The model under review builds one solid part; all positions refer to its coordinate system, in mm. A direction names the side the tool comes from. Coordinates: 2 decimals unless noted, no trailing zeros. Write each loop counter-clockwise with the first axis right and the second up, starting at its lowest first coordinate (ties: lowest second). Pieces come first, ordered by that corner, then holes. Notation, with made-up numbers: (-27.5, 37.5) - (28.5, 37.5) arc R26 cw to (28.5, 73.5) - close; hole circle Ø3 at (63, 19). An arc over 180 degrees is marked (long way). Use one line per item in the form item = value. Start each with the question number.
```python
from build123d import *

# Parameters (mm, degrees)
SKETCH1_W           = 600
SKETCH1_H           = 600
BOSS_EXTRUDE1_DEPTH = 10
SKETCH2_W           = 20
SKETCH2_H           = 60
BOSS_EXTRUDE2_DEPTH = 130
SKETCH3_W           = 600
SKETCH3_H           = 600
SKETCH3_W_2         = 20
SKETCH3_H_2         = 60
BOSS_EXTRUDE3_DEPTH = 10
SKETCH4_OUTSIDE_W   = 774
SKETCH4_OUTSIDE_H   = 774
SKETCH4_OUTSIDE_W_2 = 600
SKETCH4_OUTSIDE_H_2 = 80
CUT_EXTRUDE1_DEPTH  = 10
SKETCH5_W           = 42
SKETCH5_H           = 42
CUT_EXTRUDE2_DEPTH  = 10


with BuildPart() as part:
    # Sketch1 → Boss-Extrude1 (new body)
    with BuildSketch(Plane(origin=(0, 0, 0), x_dir=(1, 0, 0), z_dir=(0, 1, 0))):
        Rectangle(SKETCH1_W, SKETCH1_H)
    extrude(amount=BOSS_EXTRUDE1_DEPTH)

    # Sketch2 → Boss-Extrude2 (add)
    with BuildSketch(Plane(origin=(0, 10, 0), x_dir=(1, 0, 0), z_dir=(0, 1, 0))):
        with Locations((-250, 0)):
            Rectangle(SKETCH2_W, SKETCH2_H)
        with Locations((250, 0)):
            Rectangle(SKETCH2_W, SKETCH2_H)
    extrude(amount=BOSS_EXTRUDE2_DEPTH)

    # Sketch3 → Boss-Extrude3 (add)
    with BuildSketch(Plane(origin=(0, 110, 0), x_dir=(1, 0, 0), z_dir=(0, 1, 0))):
        Rectangle(SKETCH3_W, SKETCH3_H)
        with Locations((-250, 0)):
            Rectangle(SKETCH3_W_2, SKETCH3_H_2, mode=Mode.SUBTRACT)
        with Locations((250, 0)):
            Rectangle(SKETCH3_W_2, SKETCH3_H_2, mode=Mode.SUBTRACT)
    extrude(amount=BOSS_EXTRUDE3_DEPTH)

    # Sketch4 outside → Cut-Extrude1 (cut)
    with BuildSketch(Plane(origin=(0, 120, 0), x_dir=(1, 0, 0), z_dir=(0, 1, 0))):
        Rectangle(SKETCH4_OUTSIDE_W, SKETCH4_OUTSIDE_H)
        Rectangle(SKETCH4_OUTSIDE_W_2, SKETCH4_OUTSIDE_H_2, mode=Mode.SUBTRACT)
    extrude(amount=-CUT_EXTRUDE1_DEPTH, mode=Mode.SUBTRACT)

    # Sketch5 → Cut-Extrude2 (cut)
    with BuildSketch(Plane(origin=(0, 120, 0), x_dir=(1, 0, 0), z_dir=(0, 1, 0))):
        with Locations((-40, 0)):
            Rectangle(SKETCH5_W, SKETCH5_H)
        with Locations((40, 0)):
            Rectangle(SKETCH5_W, SKETCH5_H)
    extrude(amount=-CUT_EXTRUDE2_DEPTH, mode=Mode.SUBTRACT)


solid = part.part
```
1. For P1, Ø2, axis at x = 174, z = 136, coming from the +Y side; P2, Ø22, axis at y = 132.5, z = -7.5, coming from the -X side; P3, Ø22, axis at x = 246.5, y = 80.5, coming from the +Z side, all flat-tipped, find the tip position at first contact; note any pin that passes through.
2. Take a section at A-A (y = 53.5). State the section outline as (x, z) points, plus the area to 3 significant figures.
3. Take a section at B-B (x = -217.5). State the section outline as (y, z) points, plus the area to 3 significant figures.
4. For faces 4 (the flat face through (250, 59, 30)), 5 (the flat face through (260, 59, 0)), 6 (the flat face through (240, 130, 0)), 7 (the flat face through (240, 59, 0)), 8 (the flat face through (260, 130, 0)), list the 3-axis set-ups (+Z, -Z, +X, -X, +Y, -Y) from which the entire face can be reached by the end or side of a thin tool; tool diameter is ignored.
5. Take a section at C-C (z = 131). State the section outline as (x, y) points.
6. For L1, parallel to Z at x = -77.5, y = 118; L2, parallel to X at y = 75, z = 16; L3, parallel to Y at x = 233, z = 20, list the stretches that pass through material, from the lowest coordinate up.
7. The part is to be moulded in two halves that separate along Y. For faces 1 (the flat face through (250, 140, 0)), 2 (the flat face through (-250, 130, -30)), 3 (the flat face through (-260, 59, 0)), say which applies: released by +Y, released by -Y, zero draft, split by the parting line, or undercut.
Returned:
q1.P1 = 10
q1.P2 = -260
q1.P3 = 30
q2.outline = (-260, -30) - (-240, -30) - (-240, 30) - (-260, 30) - close; (240, -30) - (260, -30) - (260, 30) - (240, 30) - close
q2.area = 2,400 mm²
q3.outline = (0, -300) - (10, -300) - (10, 300) - (0, 300) - close; (110, -40) - (120, -40) - (120, 40) - (110, 40) - close
q3.area = 6,800 mm²
q4.face_4 = +Z, +X, -X
q4.face_5 = +Z, -Z, +X
q4.face_6 = +Z, -Z, +Y
q4.face_7 = +Z, -Z
q4.face_8 = +Z, -Z, +X, +Y
q5.outline = (-300, 0) - (300, 0) - (300, 10) - (-300, 10) - close
q6.L1 = -40 to 40
q6.L2 = -260 to -240, 240 to 260
q6.L3 = 0 to 10, 110 to 120
q7.face_1 = released by +Y
q7.face_2 = zero draft
q7.face_3 = undercut
